Geometry check sheet. Reference: the model listing, model coordinates, mm. Give positions to 0.01 mm unless a question says otherwise; leave off trailing zeros. Write each loop counter-clockwise with the first axis right and the second up, starting at its lowest first coordinate (ties: lowest second). Pieces come first, ordered by that corner, then holes.
(1) Cross-section at A-A (x = 37). Record the boundary of the cut face in (y, z), and give its area (3 significant figures).
(2) Depth check by flat-ended pin: P1, Ø1, axis at y = -6, z = -23, coming from the -X side; P2, Ø1, axis at x = -36, y = -5, coming from the +Z side; P3, Ø1.5, axis at y = -8, z = 15.5, coming from the -X side. Enter the tip coordinate at first touch or a pass-through.
(3) Thickness scan on line 1 along Z through (x, y) = (-36.5, -3.25); line 2 along X through (y, z) = (-20.5, 43.5); line 3 along X through (y, z) = (-2.25, -24). Record the ranges inside material, lowest first.
(4) Cross-section at D-D (x = 0). Record the boundary of the cut face in (y, z), and give its area (3 significant figures).
(5) Mould release check, pull along X, two halves, no side actions. Record for faces 1 (the cylindrical face through (-33.659, -12.325, 33.795)), 2 (the cylindrical face through (12.252, -12.325, -46.097)), 3 (the cylindrical face through (-0.119, -12.675, 42.054)): +X half, -X half, draft (parallel to the pull), parting line (faces both ways), or undercut.
(6) Cross-section at C-C (z = 0). Record the boundary of the cut face in (x, y).
(7) Cross-section at B-B (y = -15). Record the boundary of the cut face in (x, z).
```python
from build123d import *

# Parameters (mm, degrees)
F0_R            = 47.6973653994
F1_DEPTH        = 25
F3_DEPTH        = 25
F3_COPIES_COUNT = 12


# Not quite as in the source:
# - a feature of the source that left no trace in its solid (it failed there, or was rolled back) is left out
# - a pattern or mirror of a feature is missing from the dataset's text; its kind, count and spacing are read off the source's solid


with BuildPart() as f1:
    # F0 (on Front) → F1 (new body)
    with BuildSketch(Plane.XZ):
        Circle(F0_R)
    extrude(amount=F1_DEPTH)

    # F2 (on face) → F3 (cut)
    with BuildSketch(Plane.XZ.offset(25)):
        with BuildLine():
            ThreePointArc((5.635130152, 47.3633188683), (0, 47.6973653994), (-5.635130152, 47.3633188683))
            ThreePointArc((-5.635130152, 47.3633188683), (0, 42.0523429092), (5.635130152, 47.3633188683))
        make_face()
    f3 = extrude(amount=-F3_DEPTH, mode=Mode.SUBTRACT)

    # F3_copies: F3 ×12 about axis
    f3_copies_axis = Axis((0, 0, 0), (0, 1, 0))
    for i in range(1, F3_COPIES_COUNT):
        add(f3.rotate(f3_copies_axis, i * 360 / F3_COPIES_COUNT), mode=Mode.SUBTRACT)


solid = f1.part
```
Reply:
1. outline: (-25, -30.1) - (0, -30.1) - (0, -27.5) - (-25, -27.5) - close; (-25, -20.2) - (0, -20.2) - (0, 20.2) - (-25, 20.2) - close; (-25, 27.5) - (0, 27.5) - (0, 30.1) - (-25, 30.1) - close
1. area: 1,140 mm2
2. P1: stops at x = -35.83
2. P2: stops at z = 31.86
2. P3: stops at x = -45.36
3. line 1: z = -30.7 to -26.81, -20.89 to 20.89, 26.81 to 30.7
3. line 2: x = -18.65 to -3.77, 3.77 to 18.65
3. line 3: x = -35.66 to 35.66
4. outline: (-25, -42.05) - (0, -42.05) - (0, 42.05) - (-25, 42.05) - close
4. area: 2,100 mm2
5. face 1: -X half
5. face 2: +X half
5. face 3: undercut
6. outline: (-42.05, -25) - (42.05, -25) - (42.05, 0) - (-42.05, 0) - close
7. outline: (-47.36, -5.64) arc R47.7 ccw to (-43.84, -18.8) arc R5.65 cw to (-38.2, -28.56) arc R47.7 ccw to (-28.56, -38.2) arc R5.65 cw to (-18.8, -43.84) arc R47.7 ccw to (-5.64, -47.36) arc R5.65 cw to (5.64, -47.36) arc R47.7 ccw to (18.8, -43.84) arc R5.65 cw to (28.56, -38.2) arc R47.7 ccw to (38.2, -28.56) arc R5.65 cw to (43.84, -18.8) arc R47.7 ccw to (47.36, -5.64) arc R5.65 cw to (47.36, 5.64) arc R47.7 ccw to (43.84, 18.8) arc R5.65 cw to (38.2, 28.56) arc R47.7 ccw to (28.56, 38.2) arc R5.65 cw to (18.8, 43.84) arc R47.7 ccw to (5.64, 47.36) arc R5.65 cw to (-5.64, 47.36) arc R47.7 ccw to (-18.8, 43.84) arc R5.65 cw to (-28.56, 38.2) arc R47.7 ccw to (-38.2, 28.56) arc R5.65 cw to (-43.84, 18.8) arc R47.7 ccw to (-47.36, 5.64) arc R5.65 cw to start
